from build123d import *

# Parameters (mm, degrees)
BOSS_EXTRUDE1_DEPTH = 2
SKETCH2_R           = 1.75
SKETCH2_R_2         = 4
SKETCH2_R_3         = 2.25
CUT_EXTRUDE2_DEPTH  = 3
FILLET1_R           = 10
BOSS_EXTRUDE3_DEPTH = 2
FILLET3_R           = 5
SKETCH4_R           = 2.25
CUT_EXTRUDE3_DEPTH  = 3.0000001


with BuildPart() as part:
    # Sketch1 → Boss-Extrude1 (new body)
    with BuildSketch(Plane(origin=(0, 0, 0), x_dir=(1, 0, 0), z_dir=(0, 1, 0))):
        Polygon((0, 0), (0, -98.655), (130, -98.655), (130, 80.835), (142.835, 80.835), (142.835, 20.135), (155, 7.97), (155, -55.71), (165.445, -66.155), (165.445, -116.155), (-35.445, -116.155), (-35.445, -66.155), (-25, -55.71), (-25, -14.597979746), (-42.835, 3.237020254), (-42.835, 80.835), (-14.835, 80.835), (-14.835, 14.835), align=None)
    extrude(amount=BOSS_EXTRUDE1_DEPTH)

    # Sketch2 → Cut-Extrude2 (cut, through all)
    with BuildSketch(Plane(origin=(0, 2, 0), x_dir=(1, 0, 0), z_dir=(0, 1, 0))):
        with Locations((-23.178145751, 38.49185425)):
            Circle(SKETCH2_R)
        with Locations((-23.178145751, 27.178145751)):
            Circle(SKETCH2_R)
        with Locations((-34.491854249, 27.178145751)):
            Circle(SKETCH2_R)
        with Locations((-34.491854249, 38.49185425)):
            Circle(SKETCH2_R)
        with Locations((-28.835, 32.835)):
            Circle(SKETCH2_R_2)
        with Locations((137.585, -80.14)):
            Circle(SKETCH2_R_3)
        with Locations((-7.585, -80.14)):
            Circle(SKETCH2_R_3)
        with Locations((137.585, -55.945)):
            Circle(SKETCH2_R_3)
        with Locations((-7.585, -55.945)):
            Circle(SKETCH2_R_3)
        with Locations((137.585, -31.75)):
            Circle(SKETCH2_R_3)
        with Locations((-7.585, -31.75)):
            Circle(SKETCH2_R_3)
        with Locations((137.585, -7.555)):
            Circle(SKETCH2_R_3)
        with Locations((-7.585, -7.555)):
            Circle(SKETCH2_R_3)
        with Locations((16.61, -104.335)):
            Circle(SKETCH2_R_3)
        with Locations((40.805, -104.335)):
            Circle(SKETCH2_R_3)
        with Locations((65, -104.335)):
            Circle(SKETCH2_R_3)
        with Locations((89.195, -104.335)):
            Circle(SKETCH2_R_3)
        with Locations((113.39, -104.335)):
            Circle(SKETCH2_R_3)
    extrude(amount=-CUT_EXTRUDE2_DEPTH, mode=Mode.SUBTRACT)

    # Fillet1
    fillet1_edges = [part.edges().sort_by_distance(p)[0] for p in [
        (0, 1, 0),
        (142.835, 1, -20.135),
        (155, 1, -7.97),
        (155, 1, 55.71),
        (165.445, 1, 66.155),
        (165.445, 1, 116.155),
        (-35.445, 1, 116.155),
        (-35.445, 1, 66.155),
        (-25, 1, 55.71),
        (-25, 1, 14.597979746),
        (-42.835, 1, -3.237020254),
        (-42.835, 1, -80.835),
        (-14.835, 1, -80.835),
    ]]
    fillet(fillet1_edges, radius=FILLET1_R)

    # Sketch3 → Boss-Extrude3 (add, through all)
    with BuildSketch(Plane(origin=(0, 2, 0), x_dir=(1, 0, 0), z_dir=(0, 1, 0))):
        with BuildLine():
            Line((0, -18.655), (0, -98.655))
            Line((0, -98.655), (20, -98.655))
            add(Edge.make_bspline(
                [(0, -18.655), (0, -98.655), (20, -98.655)],
                knots=[4.71238898, 4.71238898, 4.71238898, 6.283185307, 6.283185307, 6.283185307], degree=2, weights=[1, 0.707106781, 1]))
        make_face()
        with BuildLine():
            Line((130, -98.655), (110, -98.655))
            add(Edge.make_bspline(
                [(110, -98.655), (130, -98.655), (130, -18.655)],
                knots=[0, 0, 0, 1.570796327, 1.570796327, 1.570796327], degree=2, weights=[1, 0.707106781, 1]))
            Line((130, -18.655), (130, -98.655))
        make_face()
    extrude(amount=-BOSS_EXTRUDE3_DEPTH)

    # Fillet3
    fillet3_edges = [part.edges().sort_by_distance(p)[0] for p in [
        (130, 1, -80.835),
        (142.835, 1, -80.835),
    ]]
    fillet(fillet3_edges, radius=FILLET3_R)

    # Sketch4 → Cut-Extrude3 (cut, through all)
    with BuildSketch(Plane(origin=(0, 2, 0), x_dir=(1, 0, 0), z_dir=(0, 1, 0))):
        with Locations((-28.835, 66.835)):
            Circle(SKETCH4_R)
    extrude(amount=-CUT_EXTRUDE3_DEPTH, mode=Mode.SUBTRACT)


solid = part.part
Verification items for the finished model (mm, model axes). A direction names the side the tool comes from. Give positions to 0.01 mm unless a question says otherwise; leave off trailing zeros. Loops run counter-clockwise (first coordinate to the right, second up) from the corner with the lowest first, then second, coordinate; pieces in that order, holes last.
1) Depth check by flat-ended pin: pin 1 Ø0.6 at (y, z) = (1.5, 83) entering from -X (3 decimals). Enter the tip coordinate at first touch or a pass-through.
2) Sectioned sample at B-B, the plane z = -21.5. Enter the section's corners in (x, y) (3 decimals).
3) Thickness scan on line 1 along Z through (x, y) = (-24.5, 1.45) (3 decimals); line 2 along X through (y, z) = (1.25, 81.5) (3 decimals); line 3 along X through (y, z) = (0.2, 30). Record the ranges inside material, lowest first.
4) Draft check along X on faces 4 (the flat face through (-33.8, 1, 5.8)), 5 (the cylindrical face through (63.21, 1.01, 105.7)), 6 (the flat face through (160.19, 0.99, 60.9)). Enter one of: pulls with the +X half, pulls with the -X half, needs draft (parallel to the pull), parting line crosses it, or undercut.
5) Set-up check for faces 1 (the flat face through (-30.25, 0.99, 60.96)), 2 (the cylindrical face through (-17.69, 1.01, -77.83)), 3 (the cylindrical face through (135.799, 1.014, 57.314)): record each of +Z, -Z, +X, -X, +Y, -Y from which the full face is reachable in a straight line by a thin tool's end or side.
6) Sectioned sample at A-A, the plane z = -57. Enter the section's corners in (x, y) (3 decimals), then the cut area to 3 significant figures.
7) Sectioned sample at C-C, the plane y = 0.7. Count the separate pieces of the cut face and the enclosed holes in it, then the cut area to 3 significant figures.
Answers:
1. pin 1: stops at x = -35.445
2. outline: (-42.835, 0) - (-14.835, 0) - (-14.835, 2) - (-42.835, 2) - close; (130, 0) - (143.228, 0) - (143.228, 2) - (130, 2) - close
3. line 1: z = -80.829 to -39.639, -37.345 to -28.325, -26.031 to 116.155
3. line 2: x = -35.445 to -9.377, -5.793 to 7.624, 122.376 to 135.793, 139.377 to 165.445
3. line 3: x = -25 to -9, -6.17 to 0.2, 129.8 to 136.17, 139 to 155
4. face 4: pulls with the -X half
4. face 5: undercut
4. face 6: pulls with the +X half
5. face 1: -X, +Y, -Y
5. face 2: -Z, +Y, -Y
5. face 3: +Y, -Y
6. outline: (-42.835, 0) - (-14.835, 0) - (-14.835, 2) - (-42.835, 2) - close; (130, 0) - (142.835, 0) - (142.835, 2) - (130, 2) - close
6. area: 81.7 mm2
7. separate pieces: 1
7. enclosed holes: 19
7. area: 13,200 mm2
